Read the model definition and answer for the solid it produces. Units are mm, in the model's axes. Face numbers are marked on the shaded views. A direction names the side the tool comes from. Coordinates: 2 decimals unless noted, no trailing zeros. Write each loop counter-clockwise with the first axis right and the second up, starting at its lowest first coordinate (ties: lowest second). Pieces come first, ordered by that corner, then holes. Notation, with made-up numbers: M 47.25,24.5 L 103.25,24.5 A12 ccw 103.25,31.5 Z; hole C -8,19.25 d2. An arc over 180 degrees is marked long. Write item = value, one per line.
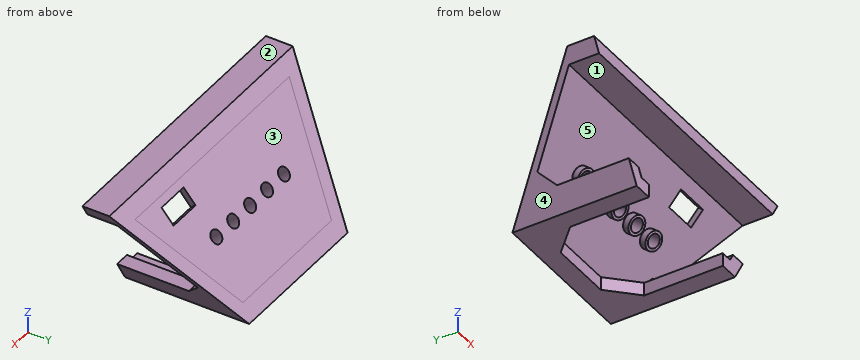
from build123d import *
from OCP.BRepFilletAPI import BRepFilletAPI_MakeChamfer

# Parameters (mm, degrees)
BOSS_EXTRUDE1_DEPTH = 10.13
BOSS_EXTRUDE2_DEPTH = 36.74
CHAMFER1_SIZE2      = 43.55
CHAMFER1_SIZE       = 36.74
CUT_EXTRUDE1_DEPTH  = 50
BOSS_EXTRUDE3_DEPTH = 3
SKETCH12_W          = 43.74
SKETCH12_H          = 39.651859931
CUT_EXTRUDE2_DEPTH  = 5
CUT_EXTRUDE3_REACH  = 127.686
SKETCH13_R          = 2.5
SKETCH15_R          = 3.5
SKETCH15_R_2        = 2.5
BOSS_EXTRUDE4_DEPTH = 5
CUT_EXTRUDE4_REACH  = 127.686
SKETCH16_W          = 13
SKETCH16_H          = 7
LPATTERN1_COUNT     = 5
LPATTERN1_PITCH     = 10
LPATTERN2_COUNT     = 5
LPATTERN2_PITCH     = 10
CUT_EXTRUDE5_REACH  = 167.082
CHAMFER2_SIZE       = 10
CHAMFER2_SIZE2      = 7.096456913
CHAMFER3_SIZE       = 10


with BuildPart() as part:
    # Sketch1 → Boss-Extrude1 (new body)
    with BuildSketch(Plane(origin=(0, 0, 0), x_dir=(1, 0, 0), z_dir=(0, 1, 0))):
        Polygon((0, 0), (108.46, 0), (83.3, 43.55), (25.16, 43.55), align=None)
    extrude(amount=BOSS_EXTRUDE1_DEPTH)

    # Sketch4 → Boss-Extrude2 (add)
    with BuildSketch(Plane(origin=(0, 10.13, 0), x_dir=(1, 0, 0), z_dir=(0, 1, 0))):
        Polygon((25.16, 43.55), (0, 0), (108.46, 0), (83.3, 43.55), align=None)
    extrude(amount=BOSS_EXTRUDE2_DEPTH)

    # Chamfer1
    chamfer1_edges = [part.edges().sort_by_distance(p)[0] for p in [
        (54.23, 46.87, 0),
    ]]
    chamfer1_side = [part.faces().sort_by_distance(p)[0] for p in [
        (54.23, 46.1352, 0),
    ]]
    chamfer(chamfer1_edges, length=CHAMFER1_SIZE - 0.0001, length2=CHAMFER1_SIZE2 - 0.0001, reference=chamfer1_side[0])  # a hair under: the kernel refuses the full size

    # Sketch10 → Cut-Extrude1 (cut)
    with BuildSketch(Plane.XZ):
        Polygon((8.66307788, -5), (28.045810372, -38.55), (80.414189628, -38.55), (99.79692212, -5), align=None)
    extrude(amount=-CUT_EXTRUDE1_DEPTH, mode=Mode.SUBTRACT)

    # Sketch11 → Boss-Extrude3 (add, along a direction that is not the sketch's normal)
    with BuildSketch(Plane(origin=(0, 5.918064684, 4.992645155), x_dir=(1, 0, 0), z_dir=(0, 0.7643374360351171, 0.6448164730179148))):
        Polygon((8.66307788, 13.073604254), (99.79692212, 13.073604254), (80.414189628, 56.967830048), (28.045810372, 56.967830048), align=None)
    extrude(amount=-BOSS_EXTRUDE3_DEPTH, dir=(0, 1, 0))

    # Sketch12 → Cut-Extrude2 (cut)
    with BuildSketch(Plane(origin=(0, 0, -43.55), x_dir=(-1, 0, 0), z_dir=(0, 0, -1))):
        with Locations((-54.23, 19.825929966)):
            Rectangle(SKETCH12_W, SKETCH12_H)
    extrude(amount=-CUT_EXTRUDE2_DEPTH, mode=Mode.SUBTRACT)

    # Sketch13 → Cut-Extrude3 (cut, up to next)
    with BuildSketch(Plane(origin=(0, 5.918064684, 4.992645155), x_dir=(1, 0, 0), z_dir=(0, 0.7643374360351171, 0.6448164730179148)), mode=Mode.PRIVATE) as cut_extrude3_sk1:
        with Locations(Location((74.23, 35.27486423, 0), (0, 0, 270))):
            Circle(SKETCH13_R)
    cut_extrude3_tool1 = extrude(cut_extrude3_sk1.sketch, amount=-CUT_EXTRUDE3_REACH, mode=Mode.PRIVATE) & part.part
    cut_extrude3 = cut_extrude3_tool1.solids().sort_by_distance((74.23, 28.663878, -21.969254))[0]
    add(cut_extrude3, mode=Mode.SUBTRACT)

    # Sketch15 → Boss-Extrude4 (add)
    with BuildSketch(Plane(origin=(0, 5.918064684, 4.992645155), x_dir=(1, 0, 0), z_dir=(0, 0.7643374360351171, 0.6448164730179148))):
        with Locations(Location((74.23, 35.27486423, 0), (0, 0, 270))):
            Circle(SKETCH15_R)
        with Locations(Location((74.23, 35.27486423, 0), (0, 0, 270))):
            Circle(SKETCH15_R_2, mode=Mode.SUBTRACT)
    boss_extrude4 = extrude(amount=-BOSS_EXTRUDE4_DEPTH)

    # Sketch16 → Cut-Extrude4 (cut, up to next)
    with BuildSketch(Plane(origin=(0, 5.918064684, 4.992645155), x_dir=(1, 0, 0), z_dir=(0, 0.7643374360351172, 0.6448164730179149)), mode=Mode.PRIVATE) as cut_extrude4_sk1:
        with Locations((80.69536615, 19.590719272)):
            Rectangle(SKETCH16_W, SKETCH16_H)
    cut_extrude4_tool1 = extrude(cut_extrude4_sk1.sketch, amount=-CUT_EXTRUDE4_REACH, mode=Mode.PRIVATE) & part.part
    add(cut_extrude4_tool1.solids().sort_by_distance((80.695366, 18.550483, -9.981275))[0], mode=Mode.SUBTRACT)

    # LPattern1: Cut-Extrude3 ×5
    with Locations(*[(-i * LPATTERN1_PITCH, 0, 0) for i in range(1, LPATTERN1_COUNT)]):
        add(cut_extrude3, mode=Mode.SUBTRACT)

    # LPattern2: Boss-Extrude4 ×5
    with Locations(*[(-i * LPATTERN2_PITCH, 0, 0) for i in range(1, LPATTERN2_COUNT)]):
        add(boss_extrude4)

    # Cut-Extrude5: up to this plane
    cut_extrude5_end = Plane(origin=(0, 0, 0), z_dir=(0, -1, 0))
    # Sketch20 → Cut-Extrude5 (cut, up to the surface)
    with BuildSketch(Plane(origin=(0, 4.165429536, 3.514073046), x_dir=(1, 0, 0), z_dir=(0, -0.7643374360351171, -0.644816473017915)), mode=Mode.PRIVATE) as cut_extrude5_sk1:
        Polygon((10.517235303, -11.139154835), (2.034423094, -11.139154835), (19.650842851, -51.033380629), (29.759813719, -51.033380629), align=None)
    cut_extrude5_tool1 = split(extrude(cut_extrude5_sk1.sketch, amount=CUT_EXTRUDE5_REACH, dir=(0, -1, 0), mode=Mode.PRIVATE), bisect_by=cut_extrude5_end, keep=Keep.BOTH, mode=Mode.PRIVATE)
    add(cut_extrude5_tool1.solids().sort_by_distance((15.759239, 24.585372, -20.690839))[0], mode=Mode.SUBTRACT)
    # Sketch20 → Cut-Extrude5 (cut, up to the surface)
    with BuildSketch(Plane(origin=(0, 4.165429536, 3.514073046), x_dir=(1, 0, 0), z_dir=(0, -0.7643374360351171, -0.644816473017915)), mode=Mode.PRIVATE) as cut_extrude5_sk2:
        Polygon((78.700186281, -51.033380629), (97.942764697, -11.139154835), (106.425576906, -11.139154835), (88.809157149, -51.033380629), align=None)
    cut_extrude5_tool2 = split(extrude(cut_extrude5_sk2.sketch, amount=CUT_EXTRUDE5_REACH, dir=(0, -1, 0), mode=Mode.PRIVATE), bisect_by=cut_extrude5_end, keep=Keep.BOTH, mode=Mode.PRIVATE)
    add(cut_extrude5_tool2.solids().sort_by_distance((92.700761, 24.585372, -20.690839))[0], mode=Mode.SUBTRACT)

    # Chamfer2: one chamfer whose edges measure the first distance from different faces: ONE call of the kernel's chamfer builder (chamfer() names one face for all edges)
    chamfer2_edges_1 = [part.edges().sort_by_distance(p)[0] for p in [
        (23.392275575, 37.072594039, -35.492650256),
    ]]
    chamfer2_side_1 = [part.faces().sort_by_distance(p)[0] for p in [
        (23.392275575, 18.53629702, -35.492650256),
    ]]
    chamfer2_edges_2 = [part.edges().sort_by_distance(p)[0] for p in [
        (85.067724425, 37.072594039, -35.492650256),
    ]]
    chamfer2_side_2 = [part.faces().sort_by_distance(p)[0] for p in [
        (85.067724425, 18.53629702, -35.492650256),
    ]]
    chamfer2 = BRepFilletAPI_MakeChamfer(part.part.solid().wrapped)
    for e in chamfer2_edges_1:
        chamfer2.Add(CHAMFER2_SIZE, CHAMFER2_SIZE2, e.wrapped, chamfer2_side_1[0].wrapped)  # the first distance lies on this face
    for e in chamfer2_edges_2:
        chamfer2.Add(CHAMFER2_SIZE, CHAMFER2_SIZE2, e.wrapped, chamfer2_side_2[0].wrapped)  # the first distance lies on this face
    add(Compound.cast(chamfer2.Shape()), mode=Mode.REPLACE)

    # Chamfer3
    chamfer3_edges = [part.edges().sort_by_distance(p)[0] for p in [
        (32.36, 39.651859931, -41.05),
        (76.1, 39.651859931, -41.05),
    ]]
    chamfer(chamfer3_edges, length=CHAMFER3_SIZE)


solid = part.part
Item 1: For a pull along X with two mould halves and no side action, classify the marked faces 3, 4 and 5 as released by +X, released by -X, zero draft, split by the parting line, or undercut.
Worked answers:
face_3 = zero draft
face_4 = released by -X
face_5 = undercut
Item 2: Consider line 1 along Z through (x, y) = (7, 6); line 2 along X through (y, z) = (2, -39.5); line 3 along X through (y, z) = (12.5, -41). Determine where each line is inside the solid, lowest interval first. Write a range as from..to.
Worked answers:
line_1 = -5..0
line_2 = 22.82..32.36, 76.1..85.64
line_3 = 23.69..32.36, 76.1..84.77
Item 3: Which of the six approach directions +Z, -Z, +X, -X, +Y, -Y give full straight-line access (tool end or side, diameter ignored) to the marked faces 1 and 2?
Worked answers:
face_1 = +X, -X, -Y
face_2 = +Z, +X, -X, +Y, -Y
Item 4: Flat-ended cylindrical pins translate along their axes: pin 1 (12 mm diameter, centred on y = 5, z = -7, fed in from -X); pin 2 (4 mm diameter, centred on y = 31.5, z = -34.5, fed in from +X); pin 3 (5 mm diameter, centred on y = 18, z = -10, fed in from +X). Find the tip coordinate at first contact, or state that the pin passes through.
Worked answers:
pin_1 = 0.58
pin_2 = 89.68
pin_3 = 103.93
Item 5: Find section A-A (y = 7.5). Determine the outline of the cut face in (x, z), and give its area (3 significant figures).
Worked answers:
outline = M 0,0 L 2.89,-5 L 105.57,-5 L 108.46,0 Z; M 20.51,-35.49 L 25.16,-43.55 L 32.36,-43.55 L 32.36,-38.55 L 28.05,-38.55 L 26.28,-35.49 Z; M 76.1,-43.55 L 83.3,-43.55 L 87.95,-35.49 L 82.18,-35.49 L 80.41,-38.55 L 76.1,-38.55 Z
area = 650 mm²
Item 6: Find section B-B (x = 102). Determine the outline of the cut face in (y, z), and give its area (3 significant figures).
Worked answers:
outline = M 0,-5 L 11.35,-5 L 16.56,-11.18 L 19.56,-11.18 L 10.13,0 L 0,0 Z
area = 79.7 mm²
